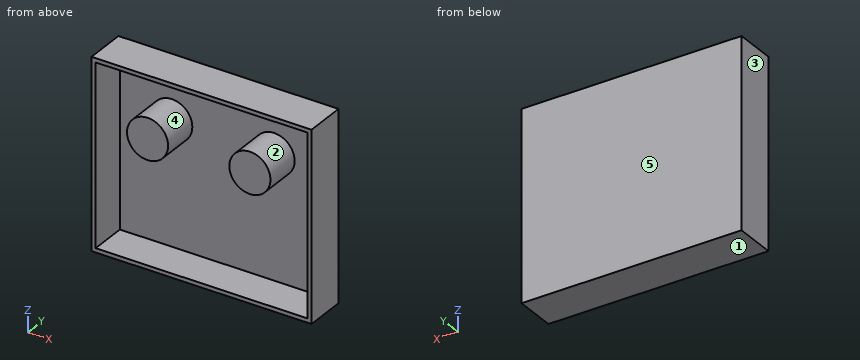
from build123d import *

# Parameters (mm, degrees)
F0_W     = 135.941163
F0_H     = 116.412658
F1_DEPTH = 25.4
F2_T     = -2.54
F3_R     = 12.7
F4_DEPTH = 25.4
F5_R     = 12.7
F6_DEPTH = 25.4


with BuildPart() as f1:
    # F0 (on Front) → F1 (new body)
    with BuildSketch(Plane.XZ):
        with Locations((-4.739925, 2.938757)):
            Rectangle(F0_W, F0_H)
    extrude(amount=F1_DEPTH)

    # F2
    f2_openings = [f1.faces().sort_by_distance(p)[0] for p in [
        (-4.739925, -25.4, 2.938757),
    ]]
    offset(amount=F2_T, openings=f2_openings)

    # F3 (on Front) → F4 (join)
    with BuildSketch(Plane.XZ):
        with Locations((-38.1, 23.045086)):
            Circle(F3_R)
    extrude(amount=F4_DEPTH)

    # F5 (on Front) → F6 (join)
    with BuildSketch(Plane.XZ):
        with Locations((25.130656, 23.045086)):
            Circle(F5_R)
    extrude(amount=F6_DEPTH)


solid = f1.part
Input: part model. Units: mm. Frame: model coordinates. Face numbers are marked on the shaded views. A direction names the side the tool comes from. Give positions to 0.01 mm unless a question says otherwise; leave off trailing zeros. Loops run counter-clockwise (first coordinate to the right, second up) from the corner with the lowest first, then second, coordinate; pieces in that order, holes last. Notation, with made-up numbers: M 76,-19.75 L 106,-19.75 A13 cw 106,-10.75 Z; hole C -20.5,22.5 d10. An arc over 180 degrees is marked long. Use CSV: the item, a comma, the result in double quotes.
(1) Material intervals for L1, parallel to X at y = -16.75, z = 54; L2, parallel to Z at x = 10.5, y = -11.25; L3, parallel to Z at x = 17, y = -9, sorted ascending. Write a range as [from, to].
Outcome:
L1,"x = [-72.71, -70.17], [60.69, 63.23]"
L2,"z = [-55.27, -52.73], [58.61, 61.15]"
L3,"z = [-55.27, -52.73], [13.29, 32.8], [58.61, 61.15]"
(2) Section A-A, the plane y = -16.75. Return loops of the section in (x, z).
Outcome:
outline,"M -72.71,-55.27 L 63.23,-55.27 L 63.23,61.15 L -72.71,61.15 Z; C -38.1,23.05 d25.4; C 25.13,23.05 d25.4; hole M -70.17,-52.73 L 60.69,-52.73 L 60.69,58.61 L -70.17,58.61 Z"
(3) Section D-D, the plane x = -3.5. Return loops of the section in (y, z), plus the area to 3 significant figures.
Outcome:
outline,"M -25.4,-55.27 L 0,-55.27 L 0,61.15 L -25.4,61.15 L -25.4,58.61 L -2.54,58.61 L -2.54,-52.73 L -25.4,-52.73 Z"
area,"412 mm²"
(4) Pull-direction query (Z, two-part tool) for the marked faces 1, 2 and 3; classes: pulls with the +Z half, pulls with the -Z half, needs draft (parallel to the pull), parting line crosses it, or undercut.
Outcome:
face 1,"pulls with the -Z half"
face 2,"undercut"
face 3,"needs draft"
(5) Set-up query: the marked faces 4 and 5. Return all of +Z, -Z, +X, -X, +Y, -Y with unobstructed straight access to the full face (end or side cutting, diameter ignored); none if empty.
Outcome:
face 4,"-Y"
face 5,"+Z, -Z, +X, -X, +Y"
(6) Pin query (flat end, axial travel): P1, Ø1.5, axis at x = -9, z = -21, coming from the -Y side. Return the tip coordinate at first contact, or that it passes through.
Outcome:
P1,"stops at y = -2.54"
(7) Section B-B, the plane x = -38.1. Return loops of the section in (y, z), plus the area to 3 significant figures.
Outcome:
outline,"M -25.4,-55.27 L 0,-55.27 L 0,61.15 L -25.4,61.15 L -25.4,58.61 L -2.54,58.61 L -2.54,35.75 L -25.4,35.75 L -25.4,10.35 L -2.54,10.35 L -2.54,-52.73 L -25.4,-52.73 Z"
area,"992 mm²"
(8) Section C-C, the plane z = 21.5. Return loops of the section in (x, y) (1 decimal).
Outcome:
outline,"M -72.7,-25.4 L -70.2,-25.4 L -70.2,-2.5 L -50.7,-2.5 L -50.7,-25.4 L -25.5,-25.4 L -25.5,-2.5 L 12.5,-2.5 L 12.5,-25.4 L 37.7,-25.4 L 37.7,-2.5 L 60.7,-2.5 L 60.7,-25.4 L 63.2,-25.4 L 63.2,0 L -72.7,0 Z"
